CAD build for the part. Positions are in the model's coordinates, mm. Face numbers are marked on the shaded views. A direction names the side the tool comes from. Round coordinates to 2 decimals unless told otherwise and drop trailing zeros. Loops run counter-clockwise (first coordinate to the right, second up) from the corner with the lowest first, then second, coordinate; pieces in that order, holes last. Notation, with made-up numbers: M -11,75.25 L 4,75.25 A16 ccw 4,95.25 Z; hole C 45.5,-10 d9. An arc over 180 degrees is marked long. One line per item, written item: value. Start each with the question number.
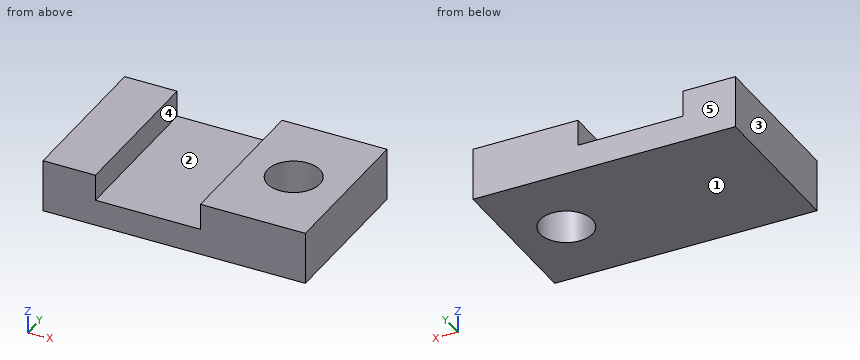
from build123d import *

# Parameters (mm, degrees)
F0_W     = 25.4
F0_H     = 76.2
F1_DEPTH = 25.4
F0_W_2   = 50.8
F2_DEPTH = 12.7
F0_R     = 12.7
F3_DEPTH = 25.4


with BuildPart() as f1:
    # F0 (on Top) → F1 (new body)
    with BuildSketch(Plane.XY):
        with Locations((-50.8, 0)):
            Rectangle(F0_W, F0_H)
    extrude(amount=F1_DEPTH)

    # F0 (on Top) → F2 (join)
    with BuildSketch(Plane.XY):
        with Locations((-12.7, 0)):
            Rectangle(F0_W_2, F0_H)
    extrude(amount=F2_DEPTH)

    # F0 (on Top) → F3 (join)
    with BuildSketch(Plane.XY):
        with Locations((38.1, 0)):
            Rectangle(F0_W_2, F0_H)
        with Locations((38.1, 0)):
            Circle(F0_R, mode=Mode.SUBTRACT)
    extrude(amount=F3_DEPTH)


solid = f1.part
(1) Mould opens along X. For the marked faces 1, 2 and 3 say: pulls with the +X half, pulls with the -X half, needs draft (parallel to the pull), parting line crosses it, or undercut.
(2) Slice it at B-B, the plane z = 21.75. List the corners of the cut face in (x, y).
(3) Probe L1, parallel to Y at x = 38.1, z = 13.5; L2, parallel to X at y = -22.5, z = 18; L3, parallel to Z at x = -18.5, y = 22.5. List the from-to ranges inside material, lowest first.
(4) Slice it at A-A, the plane x = 38.1. List the corners of the cut face in (y, z).
(5) Which spindle directions (+Z, -Z, +X, -X, +Y, -Y) get a long thin tool onto all of the face, cutting with end or side? Do the marked faces 4 and 5. Say none if no direction does.
(6) Slice it at D-D, the plane y = 28. List the corners of the cut face in (x, z).
(7) Slice it at C-C, the plane y = 0. List the corners of the cut face in (x, z).
(8) Flat gauge pins, fed straight in: P1, Ø23, axis at x = 38.1, y = 0, coming from the +Z side; P2, Ø4, axis at x = -26, y = 5, coming from the +Z side. Where does each tip first touch, or does it go through?
Check result:
1. face 1: needs draft
1. face 2: undercut
1. face 3: pulls with the -X half
2. outline: M -63.5,-38.1 L -38.1,-38.1 L -38.1,38.1 L -63.5,38.1 Z; M 12.7,-38.1 L 63.5,-38.1 L 63.5,38.1 L 12.7,38.1 Z; hole C 38.1,0 d25.4
3. L1: y = -38.1 to -12.7, 12.7 to 38.1
3. L2: x = -63.5 to -38.1, 12.7 to 63.5
3. L3: z = 0 to 12.7
4. outline: M -38.1,0 L -12.7,0 L -12.7,25.4 L -38.1,25.4 Z; M 12.7,0 L 38.1,0 L 38.1,25.4 L 12.7,25.4 Z
5. face 4: +Z, +Y, -Y
5. face 5: +Z, -Z, +X, -X, +Y
6. outline: M -63.5,0 L 63.5,0 L 63.5,25.4 L 12.7,25.4 L 12.7,12.7 L -38.1,12.7 L -38.1,25.4 L -63.5,25.4 Z
7. outline: M -63.5,0 L 25.4,0 L 25.4,25.4 L 12.7,25.4 L 12.7,12.7 L -38.1,12.7 L -38.1,25.4 L -63.5,25.4 Z; M 50.8,0 L 63.5,0 L 63.5,25.4 L 50.8,25.4 Z
8. P1: passes through
8. P2: stops at z = 12.7
